Verification items for the finished model (mm, model axes). A direction names the side the tool comes from. Coordinates: 2 decimals unless noted, no trailing zeros. Order: outer loops, then holes, each group sorted by start corner. A loop starts at its lowest first (then second) coordinate and runs counter-clockwise, first axis right, second up. Notation, with made-up numbers: M 39.25,14 L 84.25,14 A21 ccw 84.25,43 Z; hole C -17.75,53.25 d8. An arc over 180 degrees is marked long. Return JSON: item names as keys, results as strings. Group by question number.
Q1. Section check B-B, the plane x = -38. Enter the section's corners in (y, z), then the cut area to 3 significant figures.
Q2. Mould release check, pull along Y, two halves, no side actions. Record for faces 3 (the face through (56.37, -83.05, 5.89)), 4 (the face through (-29.01, 91.53, 9.87)), 5 (the face through (45.5, 56.27, 12.52)), 6 (the face through (-65.408, -30.957, 12.522)): pulls with the +Y half, pulls with the -Y half, needs draft (parallel to the pull), parting line crosses it, or undercut.
Q3. Section check C-C, the plane y = -47. Enter the section's corners in (x, z), then the cut area to 3 significant figures.
Q4. Section check A-A, the plane z = 18. Enter the section's corners in (x, y).
Q5. Go/stop test with flat-tipped pins: pin 1 Ø10 at (x, z) = (-36.5, 4.5) entering from +Y; pin 2 Ø1 at (y, z) = (-53, 18.5) entering from -X; pin 3 Ø10 at (y, z) = (19, 14) entering from +X. Record where each tip stops, or that it passes through.
Q6. Thickness scan on probe 1 along Y at (x, z) = (69, 16.75); probe 2 along Y at (x, z) = (0.5, 11.75); probe 3 along Y at (x, z) = (7, 23.5). Record the ranges inside material, lowest first.
Q7. Access from +Z, -Z, +X, -X, +Y, -Y to the whole of each face (thin tool, end or side, straight path). Record for faces 1 (the face through (80.057, -100.606, 11.937)), 2 (the face through (72.362, 0, 13)).
from build123d import *

# Parameters (mm, degrees)
F1_DEPTH = 25.4
F2_R     = 9.7144872298
F3_DEPTH = 56.2097504735
F4_R     = 8.5689068518
F5_DEPTH = 47.313503921


with BuildPart() as f1:
    # F0 (on Top) → F1 (new body)
    with BuildSketch(Plane.XY):
        Polygon((72.3621845245, -34.8477914285), (72.3621845245, 34.8477914285), (17.871983658, 78.3022765744), (-50.076185425, 62.7935503844), (-80.315965515, 0), (-50.076185425, -62.7935503844), (17.871983658, -78.3022765744), align=None)
    extrude(amount=F1_DEPTH)

    # F2 (on face) → F3 (join)
    with BuildSketch(Plane(origin=(45.1170840913, -56.5750340014, 0), x_dir=(0.7818314825, 0.6234898019, 0), z_dir=(0.6234898019, -0.7818314825, 0))):
        with Locations((0, 11.8007967249)):
            Circle(F2_R)
    extrude(amount=F3_DEPTH)

    # F4 (on face) → F5 (join)
    with BuildSketch(Plane(origin=(-16.1021008835, 70.5479134794, 0), x_dir=(-0.9749279122, -0.222520934, 0), z_dir=(-0.222520934, 0.9749279122, 0))):
        with Locations((0, 13.1539618596)):
            Circle(F4_R)
    extrude(amount=F5_DEPTH)


solid = f1.part
Numbers:
{
 "1": {"outline": "M -65.55,0 L 65.55,0 L 65.55,25.4 L -65.55,25.4 Z", "area": "3,330 mm2"},
 "2": {"face 3": "undercut", "face 4": "undercut", "face 5": "pulls with the +Y half", "face 6": "pulls with the -Y half"},
 "3": {"outline": "M -57.68,0 L 57.12,0 L 57.12,25.4 L -57.68,25.4 Z", "area": "2,920 mm2"},
 "4": {"outline": "M -80.32,0 L -50.08,-62.79 L 17.87,-78.3 L 39.27,-61.24 L 74.32,-105.18 L 86.01,-95.86 L 50.96,-51.91 L 72.36,-34.85 L 72.36,34.85 L 17.87,78.3 L -9.21,72.12 L -19.74,118.25 L -33.52,115.1 L -22.99,68.98 L -50.08,62.79 Z"},
 "5": {"pin 1": "stops at y = 115.47", "pin 2": "stops at x = -55.03", "pin 3": "stops at x = 72.36"},
 "6": {"probe 1": "y = -99.93 to -73.12, -37.53 to 37.53", "probe 2": "y = -74.34 to 74.34", "probe 3": "y = -75.82 to 75.82"},
 "7": {"face 1": "+Z, -Z, +X, -Y", "face 2": "+Z, -Z, +X, +Y"}
}
